Geometry: final body of the model. Coordinates: model frame, mm. A direction names the side the tool comes from. Give positions to 0.01 mm unless a question says otherwise; leave off trailing zeros. Write each loop counter-clockwise with the first axis right and the second up, starting at its lowest first coordinate (ties: lowest second). Pieces come first, ordered by that corner, then holes.
Q1. Cut plane B-B on x = 0. Return the cut outline in (y, z).
Q2. Cut plane A-A on y = 0. Return the cut outline in (x, z), plus the area to 3 significant figures.
Q3. Cut plane D-D on y = -32.5. Return the cut outline in (x, z), plus the area to 3 significant figures.
Q4. Pin query (flat end, axial travel): pin 1 (16 mm diameter, centred on x = -32.5, y = 0, fed in from -Z); pin 2 (2 mm diameter, centred on y = -58, z = -7, fed in from -X); pin 3 (10 mm diameter, centred on x = -42, z = 5, fed in from +Y); pin 4 (2 mm diameter, centred on x = 4.5, z = -6.5, fed in from -Y). Return the tip coordinate at first contact, or that it passes through.
Q5. Draft query along X for faces 1 (the face through (49.66, 10.27, 0.06)), 2 (the face through (0.382, 8.218, 6.958)), 3 (the face through (-22.188, -34.988, -6.958)). Return one class per face: pulls with the +X half, pulls with the -X half, needs draft (parallel to the pull), parting line crosses it, or undercut.
Q6. Line query: L1, parallel to X at y = 4, z = -1.25; L2, parallel to Y at x = -28, z = 1.5; L3, parallel to Y at x = 34.5, z = 2.25. Output: solid intervals per line, ascending.
Q7. Reachability of faces 4 (the face through (23, -36, 4)), 5 (the face through (21.8, -35.76, -6.96)), 6 (the face through (0, -80, 7)), 7 (the face through (21.8, -35.76, 6.96)), 8 (the face through (23, -36, -4)) from +Z, -Z, +X, -X, +Y, -Y: full face, straight path, thin tool, end or side. Return the list, or none.
Q8. Cut plane C-C on z = 6.25. Return the cut outline in (x, y).
```python
from build123d import *

# Parameters (mm, degrees)
SKETCH1_R           = 10
SKETCH1_R_2         = 15
BOSS_EXTRUDE1_DEPTH = 10
BOSS_EXTRUDE3_DEPTH = 4


with BuildPart() as part:
    # Sketch1 → Boss-Extrude1 (new, symmetric)
    # profile 1 of 2: a face of its own
    with BuildSketch(Plane.XY):
        with BuildLine():
            ThreePointArc((15, -65), (21.994198596, -35.372099298), (41.5, -12))
            ThreePointArc((41.5, -12), (45.460955309, 7.550737546), (26.5, 13.747727085))
            ThreePointArc((26.5, 13.747727085), (0, 8.216855043), (-26.5, 13.747727085))
            ThreePointArc((-26.5, 13.747727085), (-45.460955309, 7.550737546), (-41.5, -12))
            ThreePointArc((-41.5, -12), (-21.994198596, -35.372099298), (-15, -65))
            ThreePointArc((-15, -65), (0, -50), (15, -65))
        make_face()
        with Locations((-32.5, 0)):
            Circle(SKETCH1_R, mode=Mode.SUBTRACT)
        with Locations((32.5, 0)):
            Circle(SKETCH1_R, mode=Mode.SUBTRACT)
    # profile 2 of 2: a face of its own
    with BuildSketch(Plane.XY):
        with Locations((0, -65)):
            Circle(SKETCH1_R_2)
        with Locations((0, -65)):
            Circle(SKETCH1_R, mode=Mode.SUBTRACT)
    extrude(amount=BOSS_EXTRUDE1_DEPTH, both=True)

    # Sketch1_4 → Boss-Extrude3 (add, symmetric)
    with BuildSketch(Plane.XY):
        with BuildLine():
            ThreePointArc((-32.5, 20), (-49.513016167, 10.514622242), (-50.38854382, -8.94427191))
            Line((-50.38854382, -8.94427191), (-17.88854382, -73.94427191))
            ThreePointArc((-17.88854382, -73.94427191), (0, -85), (17.88854382, -73.94427191))
            Line((17.88854382, -73.94427191), (50.38854382, -8.94427191))
            ThreePointArc((50.38854382, -8.94427191), (49.513016167, 10.514622242), (32.5, 20))
            Line((32.5, 20), (-32.5, 20))
        make_face()
        with BuildLine():
            ThreePointArc((26.5, 13.747727085), (45.460955309, 7.550737546), (41.5, -12))
            ThreePointArc((41.5, -12), (21.994198596, -35.372099298), (15, -65))
            ThreePointArc((15, -65), (0, -80), (-15, -65))
            ThreePointArc((-15, -65), (-21.994198596, -35.372099298), (-41.5, -12))
            ThreePointArc((-41.5, -12), (-45.460955309, 7.550737546), (-26.5, 13.747727085))
            ThreePointArc((-26.5, 13.747727085), (0, 8.216855043), (26.5, 13.747727085))
        make_face(mode=Mode.SUBTRACT)
    extrude(amount=BOSS_EXTRUDE3_DEPTH, both=True)


solid = part.part
```
Data:
1. outline: (-85, -4) - (-80, -4) - (-80, -10) - (-75, -10) - (-75, 10) - (-80, 10) - (-80, 4) - (-85, 4) - close; (-55, -10) - (8.22, -10) - (8.22, -4) - (20, -4) - (20, 4) - (8.22, 4) - (8.22, 10) - (-55, 10) - close
2. outline: (-52.5, -4) - (-47.5, -4) - (-47.5, -10) - (-42.5, -10) - (-42.5, 10) - (-47.5, 10) - (-47.5, 4) - (-52.5, 4) - close; (-22.5, -10) - (22.5, -10) - (22.5, 10) - (-22.5, 10) - close; (42.5, -10) - (47.5, -10) - (47.5, -4) - (52.5, -4) - (52.5, 4) - (47.5, 4) - (47.5, 10) - (42.5, 10) - close
2. area: 1,180 mm2
3. outline: (-38.61, -4) - (-23.52, -4) - (-23.52, -10) - (23.52, -10) - (23.52, -4) - (38.61, -4) - (38.61, 4) - (23.52, 4) - (23.52, 10) - (-23.52, 10) - (-23.52, 4) - (-38.61, 4) - close
3. area: 1,180 mm2
4. pin 1: passes through
4. pin 2: stops at x = -15.48
4. pin 3: stops at y = 19.46
4. pin 4: stops at y = -79.59
5. face 1: pulls with the +X half
5. face 2: undercut
5. face 3: pulls with the -X half
6. L1: x = -52.1 to -41.67, -23.33 to 23.33, 41.67 to 52.1
6. L2: y = -53.72 to -8.93, 8.93 to 20
6. L3: y = -40.72 to -9.8, 9.8 to 19.9
7. face 4: +Z
7. face 5: -Z, +X, -Y
7. face 6: +Z, -Y
7. face 7: +Z, +X, -Y
7. face 8: -Z
8. outline: (-41.5, -12) arc R66.25 cw to (-15, -65) arc R15 ccw to (15, -65) arc R66.25 cw to (41.5, -12) arc R15 ccw to (26.5, 13.75) arc R66.25 cw to (-26.5, 13.75) arc R15 ccw to start; hole circle Ø20 at (-32.5, 0); hole circle Ø20 at (0, -65); hole circle Ø20 at (32.5, 0)
